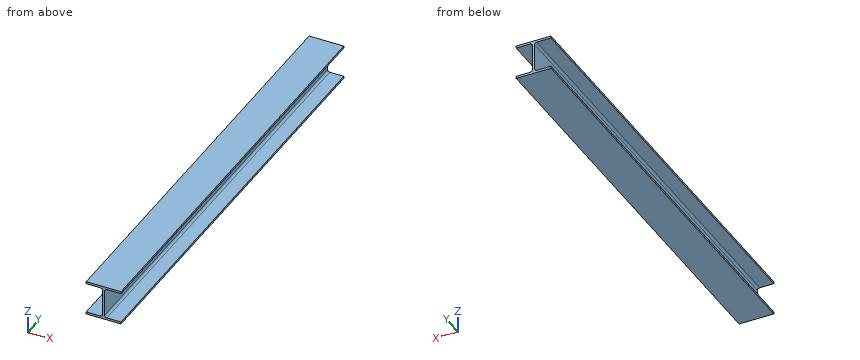
```python
from build123d import *

# Parameters (mm, degrees)
F1_DEPTH = 1270


with BuildPart() as f1:
    # F0 (on Front) → F1 (new body)
    with BuildSketch(Plane.XZ):
        with BuildLine():
            Line((50.8, 50.8), (0, 50.8))
            Line((0, 50.8), (-50.8, 50.8))
            Line((-50.8, 50.8), (-50.8, 44.45))
            Line((-50.8, 44.45), (-9.525, 44.45))
            ThreePointArc((-9.525, 44.45), (-5.034872, 42.590128), (-3.175, 38.1))
            Line((-3.175, 38.1), (-3.175, 0))
            Line((-3.175, 0), (-3.175, -38.1))
            ThreePointArc((-3.175, -38.1), (-5.034872, -42.590128), (-9.525, -44.45))
            Line((-9.525, -44.45), (-50.8, -44.45))
            Line((-50.8, -44.45), (-50.8, -50.8))
            Line((-50.8, -50.8), (0, -50.8))
            Line((0, -50.8), (50.8, -50.8))
            Line((50.8, -50.8), (50.8, -44.45))
            Line((50.8, -44.45), (9.525, -44.45))
            ThreePointArc((9.525, -44.45), (5.034872, -42.590128), (3.175, -38.1))
            Line((3.175, -38.1), (3.175, 0))
            Line((3.175, 0), (3.175, 38.1))
            ThreePointArc((3.175, 38.1), (5.034872, 42.590128), (9.525, 44.45))
            Line((9.525, 44.45), (50.8, 44.45))
            Line((50.8, 44.45), (50.8, 50.8))
        make_face()
    extrude(amount=F1_DEPTH)


solid = f1.part
```
The listing builds one solid part. Answer for the finished solid, in the listing's coordinates (mm). Give positions to 0.01 mm unless a question says otherwise; leave off trailing zeros. Loops run counter-clockwise (first coordinate to the right, second up) from the corner with the lowest first, then second, coordinate; pieces in that order, holes last. Notation, with made-up numbers: (15, 71) - (33, 71) arc R14 cw to (33, 81) - close; hole circle Ø4 at (-17.5, 44). An arc over 180 degrees is marked (long way). Answer as CSV lines item,"result". Start each with the question number.
Item 1: A cutting plane is placed at A-A on x = 28.5. Determine the outline of the cut face in (y, z).
Item 2: Find the intervals of material crossed by line 1 (Z direction, x = 12, y = -488); line 2 (X direction, y = -1097.5, z = -2) (3 decimals); line 3 (Z direction, x = 6.5, y = -312.5), in increasing order. Write a range as from..to.
Item 3: Each of these flat-tipped pins is pushed along its axis until it touches: pin 1 (3 mm diameter, centred on y = -311.5, z = -22, fed in from -X) (3 decimals); pin 2 (12 mm diameter, centred on x = 5, z = 23.5, fed in from +Y). Where does it stop, or does it pass through?
Item 4: A cutting plane is placed at B-B on y = -491.5. Determine the outline of the cut face in (x, z) (3 decimals), then the cut area to 3 significant figures.
Item 5: A cutting plane is placed at C-C on z = -13.5. Determine the outline of the cut face in (x, y) (3 decimals), then the cut area to 3 significant figures.
Found:
1,outline,"(-1270, -50.8) - (0, -50.8) - (0, -44.45) - (-1270, -44.45) - close; (-1270, 44.45) - (0, 44.45) - (0, 50.8) - (-1270, 50.8) - close"
2,line 1,"z = -50.8..-44.45, 44.45..50.8"
2,line 2,"x = -3.175..3.175"
2,line 3,"z = -50.8..-43.68, 43.68..50.8"
3,pin 1,"stops at x = -3.175"
3,pin 2,"stops at y = 0"
4,outline,"(-50.8, -50.8) - (50.8, -50.8) - (50.8, -44.45) - (9.525, -44.45) arc R6.35 cw to (3.175, -38.1) - (3.175, 38.1) arc R6.35 cw to (9.525, 44.45) - (50.8, 44.45) - (50.8, 50.8) - (-50.8, 50.8) - (-50.8, 44.45) - (-9.525, 44.45) arc R6.35 cw to (-3.175, 38.1) - (-3.175, -38.1) arc R6.35 cw to (-9.525, -44.45) - (-50.8, -44.45) - close"
4,area,"1,890 mm^2"
5,outline,"(-3.175, -1270) - (3.175, -1270) - (3.175, 0) - (-3.175, 0) - close"
5,area,"8,060 mm^2"
